from build123d import *

# Parameters (mm, degrees)
SKETCH1_R           = 2
BOSS_EXTRUDE1_DEPTH = 5


with BuildPart() as part:
    # Sketch1 → Boss-Extrude1 (new body)
    with BuildSketch(Plane(origin=(0, 0, 0), x_dir=(1, 0, 0), z_dir=(0, 1, 0))):
        with BuildLine():
            Line((-228.663769869, 10), (-118.663769869, 10))
            Line((-118.663769869, 10), (21.336230131, 10))
            Line((21.336230131, 10), (21.336230131, -106))
            Line((21.336230131, -106), (21.336230131, -136))
            Line((21.336230131, -136), (-118.663769869, -136))
            Line((-118.663769869, -136), (-228.663769869, -136))
            Line((-228.663769869, -136), (-228.663769869, -106))
            Line((-228.663769869, -106), (-124.517389937, -106))
            ThreePointArc((-124.517389937, -106), (-27.594389025, -63), (-124.517389937, -20))
            Line((-124.517389937, -20), (-228.663769869, -20))
            Line((-228.663769869, -20), (-228.663769869, 10))
        make_face()
        with Locations(Location((7.336230131, -63, 0), (0, 0, 270))):
            Circle(SKETCH1_R, mode=Mode.SUBTRACT)
        with Locations(Location((7.336230131, -43, 0), (0, 0, 270))):
            Circle(SKETCH1_R, mode=Mode.SUBTRACT)
        with Locations(Location((7.336230131, -83, 0), (0, 0, 270))):
            Circle(SKETCH1_R, mode=Mode.SUBTRACT)
    extrude(amount=BOSS_EXTRUDE1_DEPTH)


solid = part.part
Here's how the part is built. I have some questions about the finished solid (model axes, mm). A direction names the side the tool comes from. Coordinates: 2 decimals unless noted, no trailing zeros. Loops run counter-clockwise (first coordinate to the right, second up) from the corner with the lowest first, then second, coordinate; pieces in that order, holes last. Notation, with made-up numbers: (-33, 86.25) -> (6, 86.25) arc R5 cw to (6, 95.25) -> close; hole circle Ø10 at (75, 18.5). An arc over 180 degrees is marked (long way). Use one line per item in the form item = value. Start each with the question number.
(1) If we section it at C-C (z = 27.5): Please give me the cut outline in (x, y), then the cut area to 3 significant figures.
(2) We'd pull the mould along X, two halves only. Please class faces 3 (the face through (21.336, 2, 62)), 4 (the face through (-27.625, 2.465, 64.873)), 5 (the face through (-46, 5, 13)), 6 (the face through (-228.664, 2, 121)): pulls with the +X half, pulls with the -X half, needs draft (parallel to the pull), parting line crosses it, or undercut.
(3) If we section it at D-D (x = -87.5): Please give me the cut outline in (y, z).
(4) If we section it at B-B (y = 1.3): Please give me the cut outline in (x, z), then the cut area to 3 significant figures.
(5) On a 3-axis mill with a long thin cutter (end or side, diameter ignored), from which of +Z, -Z, +X, -X, +Y, -Y can I reach the whole of each face in a straight line? I mean faces 1 (the face through (-228.664, 2, 5)), 2 (the face through (-176, 2, 20)). Say none if no direction works.
(6) If we section it at A-A (x = -152): Please give me the cut outline in (y, z), then the cut area to 3 significant figures.
(7) Will this pin go through, and if not, where does the flat tip stop? pin 1 (5 mm diameter, centred on x = 7.34, z = 43, fed in from +Y).
(8) Please list where these lines run through material, in increasing order: line 1 along Z through (x, y) = (-158.5, 3.1); line 2 along X through (y, z) = (3.55, 83); line 3 along Z through (x, y) = (-114, 1.8).
Verdict:
q1.outline = (-39.73, 0) -> (21.34, 0) -> (21.34, 5) -> (-39.73, 5) -> close
q1.area = 305 mm²
q2.face_3 = pulls with the +X half
q2.face_4 = undercut
q2.face_5 = needs draft
q2.face_6 = pulls with the -X half
q3.outline = (0, -10) -> (5, -10) -> (5, 5.03) -> (0, 5.03) -> close; (0, 120.97) -> (5, 120.97) -> (5, 136) -> (0, 136) -> close
q4.outline = (-228.66, -10) -> (21.34, -10) -> (21.34, 136) -> (-228.66, 136) -> (-228.66, 106) -> (-124.52, 106) arc R58 cw (long way) to (-124.52, 20) -> (-228.66, 20) -> close; hole circle Ø4 at (7.34, 43); hole circle Ø4 at (7.34, 63); hole circle Ø4 at (7.34, 83)
q4.area = 18,100 mm²
q5.face_1 = +Z, -Z, -X, +Y, -Y
q5.face_2 = -X, +Y, -Y
q6.outline = (0, -10) -> (5, -10) -> (5, 20) -> (0, 20) -> close; (0, 106) -> (5, 106) -> (5, 136) -> (0, 136) -> close
q6.area = 300 mm²
q7.pin_1 = 5
q8.line_1 = -10 to 20, 106 to 136
q8.line_2 = -31.15 to 5.34, 9.34 to 21.34
q8.line_3 = -10 to 12.43, 113.57 to 136
